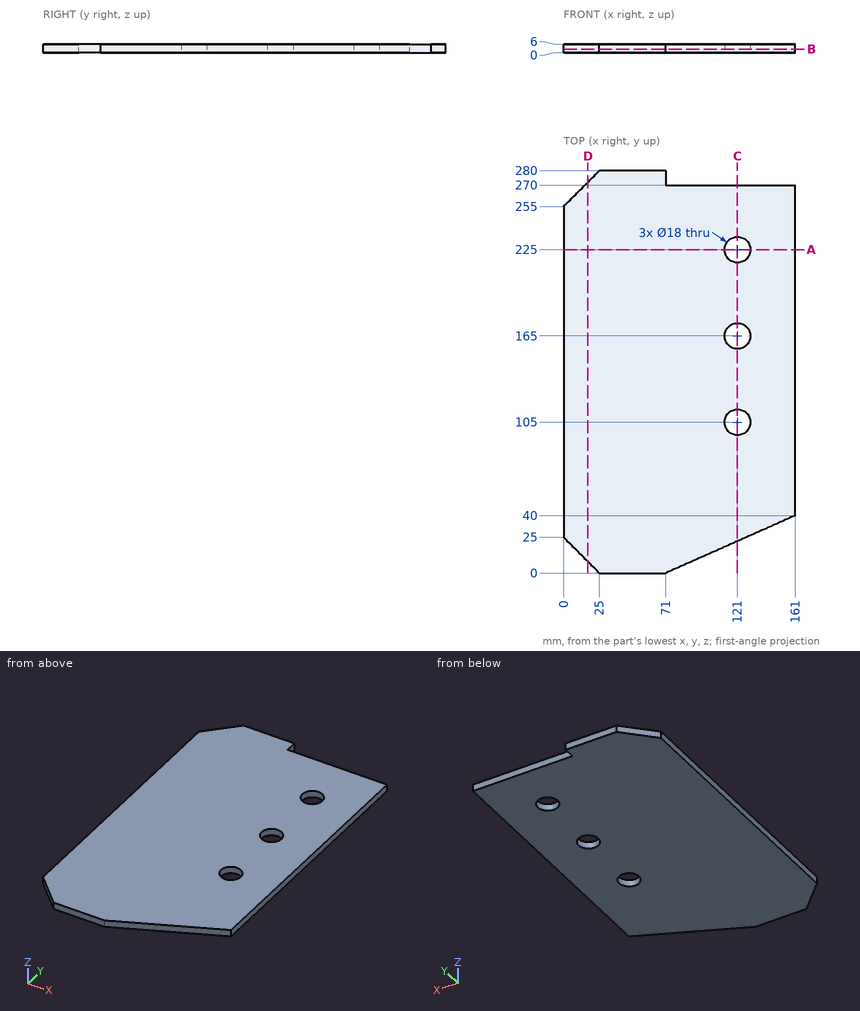
Design review of the part shown in the three views and the two pictorial views. Dimensions are in mm from the part's minimum x, y and z. Give positions to 0.01 mm unless a question says otherwise; leave off trailing zeros. Loops run counter-clockwise (first coordinate to the right, second up) from the corner with the lowest first, then second, coordinate; pieces in that order, holes last. Notation, with made-up numbers: (-27, 68.5) - (-16, 68.5) arc R21 ccw to (-16, 91.5) - close; hole circle Ø5 at (-19, -29). An arc over 180 degrees is marked (long way). Write item = value, one per line.
1) Clearance check with flat-ended pins moving along their axes: pin 1 Ø3 at (x, z) = (127.5, 4.5) entering from +Y; pin 2 Ø3 at (x, z) = (20.5, 4.5) entering from +Y; pin 3 Ø3 at (x, z) = (119.5, 1) entering from -Y. State where each tip first meets the part, or that it passes through.
Result sheet:
pin_1 = 270
pin_2 = 277
pin_3 = 20.89
2) Take a section at C-C on x = 121. State the section outline as (y, z) points.
Result sheet:
outline = (22.22, 0) - (96, 0) - (96, 6) - (22.22, 6) - close; (114, 0) - (156, 0) - (156, 6) - (114, 6) - close; (174, 0) - (216, 0) - (216, 6) - (174, 6) - close; (234, 0) - (270, 0) - (270, 6) - (234, 6) - close
3) To check wall thickness, follow line 1 (X direction, y = 225, z = 2.3); line 2 (Y direction, x = 124, z = 5.6); line 3 (Y direction, x = 121, z = 3.2). State the ranges of each line that lie inside material, in increasing order.
Result sheet:
line_1 = 0 to 112, 130 to 161
line_2 = 23.56 to 96.51, 113.49 to 156.51, 173.49 to 216.51, 233.49 to 270
line_3 = 22.22 to 96, 114 to 156, 174 to 216, 234 to 270
4) Take a section at A-A on y = 225. State the section outline as (x, z) points.
Result sheet:
outline = (0, 0) - (112, 0) - (112, 6) - (0, 6) - close; (130, 0) - (161, 0) - (161, 6) - (130, 6) - close
5) Take a section at B-B on z = 2.4. State the section outline as (x, y) points, and give its area (3 significant figures).
Result sheet:
outline = (0, 25) - (25, 0) - (71, 0) - (161, 40) - (161, 270) - (71, 270) - (71, 280) - (25, 280) - (0, 255) - close; hole circle Ø18 at (121, 105); hole circle Ø18 at (121, 165); hole circle Ø18 at (121, 225)
area = 41,000 mm2
6) Take a section at D-D on x = 17. State the section outline as (y, z) points.
Result sheet:
outline = (8, 0) - (272, 0) - (272, 6) - (8, 6) - close
